from build123d import *

# Parameters (mm, degrees)
F0_R     = 7.62
F0_R_2   = 3.2258
F1_DEPTH = 2.38125
F2_R     = 1.3843
F3_DEPTH = 7.62
F4_R     = 0.508


with BuildPart() as f1:
    # F0 (on Top) → F1 (new body, symmetric)
    with BuildSketch(Plane.XY):
        Circle(F0_R)
        Circle(F0_R_2, mode=Mode.SUBTRACT)
    extrude(amount=F1_DEPTH, both=True)

    # F2 (on Front) → F3 (cut)
    with BuildSketch(Plane.XZ):
        Circle(F2_R)
    extrude(amount=-F3_DEPTH, mode=Mode.SUBTRACT)

    # F4
    f4_edges = [f1.edges().sort_by_distance(p)[0] for p in [
        (-7.62, 0, 2.38125),
        (-7.62, 0, -2.38125),
        (-3.2258, 0, -2.38125),
        (-3.2258, 0, 2.38125),
    ]]
    fillet(f4_edges, radius=F4_R)


solid = f1.part
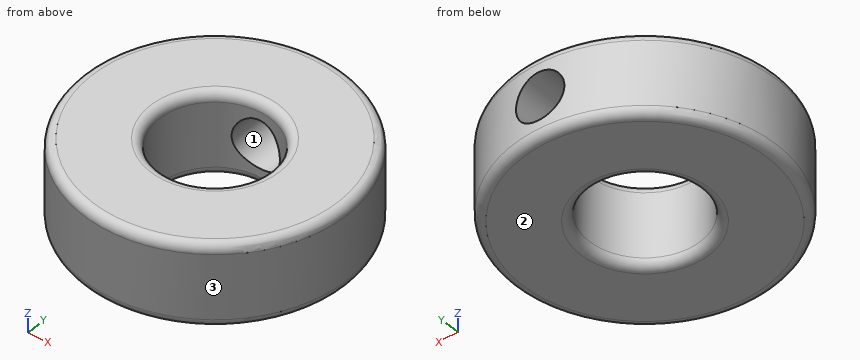
Can you work these out from the model? Positions are in its coordinate system, mm. Face numbers are marked on the shaded views. Coordinates: 2 decimals unless noted, no trailing zeros. Write each loop counter-clockwise with the first axis right and the second up, starting at its lowest first coordinate (ties: lowest second). Pieces come first, ordered by that corner, then holes. Notation, with made-up numbers: (86, -25) -> (133, -25) arc R11 cw to (133, -14) -> close; hole circle Ø6 at (27, 44.5). An arc over 180 degrees is marked (long way). Write each question's results on one line, items separated by ' | '. Start each with the question number.
Q1. We'd pull the mould along X, two halves only. Please class the marked faces 1, 2 and 3: +X half, -X half, draft (parallel to the pull), parting line (faces both ways), or undercut.
Q2. Imagine slicing it at A-A (x = 0). Write out the boundary of the cut face in (y, z), then the cut area to 3 significant figures.
Q3. Imagine slicing it at B-B (y = 0). Write out the boundary of the cut face in (x, z), then the cut area to 3 significant figures.
Q4. Imagine slicing it at C-C (z = 0). Write out the boundary of the cut face in (x, y), then the cut area to 3 significant figures.
Q5. If I drill on probe 1 along Z at (x, y) = (0, 6.3); probe 2 along Y at (x, z) = (0, 0.55); probe 3 along X at (y, z) = (5.1, 0), over which ranges is the centre line in solid material (lowest first)?
Taken from the geometry:
1) face 1: undercut | face 2: draft | face 3: parting line
2) outline: (-7.62, -1.87) arc R0.51 ccw to (-7.11, -2.38) -> (-3.73, -2.38) arc R0.51 ccw to (-3.23, -1.87) -> (-3.23, 1.87) arc R0.51 ccw to (-3.73, 2.38) -> (-7.11, 2.38) arc R0.51 ccw to (-7.62, 1.87) -> close; (3.23, -1.87) arc R0.51 ccw to (3.73, -2.38) -> (7.11, -2.38) arc R0.51 ccw to (7.62, -1.87) -> (7.62, -1.38) -> (3.23, -1.38) -> close; (3.23, 1.38) -> (7.62, 1.38) -> (7.62, 1.87) arc R0.51 ccw to (7.11, 2.38) -> (3.73, 2.38) arc R0.51 ccw to (3.23, 1.87) -> close | area: 29.2 mm^2
3) outline: (-7.62, -1.87) arc R0.51 ccw to (-7.11, -2.38) -> (-3.73, -2.38) arc R0.51 ccw to (-3.23, -1.87) -> (-3.23, 1.87) arc R0.51 ccw to (-3.73, 2.38) -> (-7.11, 2.38) arc R0.51 ccw to (-7.62, 1.87) -> close; (3.23, -1.87) arc R0.51 ccw to (3.73, -2.38) -> (7.11, -2.38) arc R0.51 ccw to (7.62, -1.87) -> (7.62, 1.87) arc R0.51 ccw to (7.11, 2.38) -> (3.73, 2.38) arc R0.51 ccw to (3.23, 1.87) -> close | area: 41.4 mm^2
4) outline: (-1.38, 2.91) -> (-1.38, 7.49) arc R7.62 ccw (long way) to (1.38, 7.49) -> (1.38, 2.91) arc R3.23 cw (long way) to start | area: 137 mm^2
5) probe 1: z = -2.38 to -1.38, 1.38 to 2.38 | probe 2: y = -7.62 to -3.23 | probe 3: x = -5.66 to -1.38, 1.38 to 5.66
